from build123d import *

# Parameters (mm, degrees)
EXTRUDE_1_DEPTH          = 50
SHELL_1_T                = -1.5
CUT_EXTRUDE_1_DEPTH      = 156.758548301
CUT_EXTRUDE_1_DEPTH_BACK = 156.758548301
SKETCH_4_R               = 3.6
SKETCH_4_R_2             = 1.6
CUT_EXTRUDE_2_REACH      = 189.083
SKETCH_6_R               = 6
SKETCH_7_R               = 1.6
CUT_EXTRUDE_3_DEPTH      = 156.758548301


with BuildPart() as part:
    # 草圖3 → 填料-伸長1 (new body)
    with BuildSketch(Plane(origin=(0, 0, 0), x_dir=(1, 0, 0), z_dir=(0, 1, 0))):
        with BuildLine():
            Line((10, 41.553121903), (90, 41.553121903))
            ThreePointArc((90, 41.553121903), (97.071067812, 38.624189715), (100, 31.553121903))
            Line((100, 31.553121903), (100, -98.446878097))
            ThreePointArc((100, -98.446878097), (97.071067812, -105.517945908), (90, -108.446878097))
            Line((90, -108.446878097), (10, -108.446878097))
            ThreePointArc((10, -108.446878097), (2.928932188, -105.517945908), (0, -98.446878097))
            Line((0, -98.446878097), (0, 31.553121903))
            ThreePointArc((0, 31.553121903), (2.928932188, 38.624189715), (10, 41.553121903))
        make_face()
    extrude(amount=EXTRUDE_1_DEPTH)

    # 薄殼1
    shell_1_openings = [part.faces().sort_by_distance(p)[0] for p in [
        (50, 50, 33.446878097),
    ]]
    offset(amount=SHELL_1_T, openings=shell_1_openings, kind=Kind.INTERSECTION)

    # 草圖4 → 除料-伸長1 (cut, two sides: drawn at the far end of the back side and taken through both)
    with BuildSketch(Plane.ZY.offset(-CUT_EXTRUDE_1_DEPTH_BACK)):
        with Locations((-6.553121903, 17)):
            Circle(SKETCH_4_R)
        with Locations((73.446878097, 17)):
            Circle(SKETCH_4_R)
        with Locations((-6.552300072, 25.5)):
            Circle(SKETCH_4_R_2)
        with Locations((-6.552300072, 8.5)):
            Circle(SKETCH_4_R_2)
        with Locations((73.447699928, 25.5)):
            Circle(SKETCH_4_R_2)
        with Locations((73.447699928, 8.5)):
            Circle(SKETCH_4_R_2)
    extrude(amount=CUT_EXTRUDE_1_DEPTH + CUT_EXTRUDE_1_DEPTH_BACK, mode=Mode.SUBTRACT)

    # 草圖6 → 除料-伸長2 (cut, up to next)
    with BuildSketch(Plane.XY.offset(108.446878097), mode=Mode.PRIVATE) as cut_extrude_2_sk1:
        with Locations((50, 35)):
            Circle(SKETCH_6_R)
    cut_extrude_2_tool1 = extrude(cut_extrude_2_sk1.sketch, amount=-CUT_EXTRUDE_2_REACH, mode=Mode.PRIVATE) & part.part
    # 草圖6 → 除料-伸長2 (cut, up to next)
    with BuildSketch(Plane.XY.offset(108.446878097), mode=Mode.PRIVATE) as cut_extrude_2_sk2:
        with Locations((50, 15)):
            Circle(SKETCH_6_R)
    cut_extrude_2_tool2 = extrude(cut_extrude_2_sk2.sketch, amount=-CUT_EXTRUDE_2_REACH, mode=Mode.PRIVATE) & part.part
    add(cut_extrude_2_tool1.solids().sort_by_distance((50, 35, 108.446878))[0], mode=Mode.SUBTRACT)
    add(cut_extrude_2_tool2.solids().sort_by_distance((50, 15, 108.446878))[0], mode=Mode.SUBTRACT)

    # 草圖7 → 除料-伸長3 (cut, through all)
    with BuildSketch(Plane(origin=(100, 0, 0), x_dir=(0, 0, -1), z_dir=(1, 0, 0))):
        with Locations((-88.446878097, 46)):
            Circle(SKETCH_7_R)
        with Locations((21.553121903, 46)):
            Circle(SKETCH_7_R)
    extrude(amount=-CUT_EXTRUDE_3_DEPTH, mode=Mode.SUBTRACT)


solid = part.part
For this review, take the finished solid that the model builds, in its own axes (mm). A direction names the side the tool comes from. Give positions to 0.01 mm unless a question says otherwise; leave off trailing zeros. Loops run counter-clockwise (first coordinate to the right, second up) from the corner with the lowest first, then second, coordinate; pieces in that order, holes last. Notation, with made-up numbers: M 4,50 L 47,50 A31 cw 47,89 Z; hole C 50,-0.5 d3. An arc over 180 degrees is marked long. Answer as a JSON object with one key per item and string values. Group by question number.
Q1. For probe 1 along Z at (x, y) = (25, 24.5); probe 2 along X at (y, z) = (15.5, 32.5); probe 3 along Y at (x, z) = (30.5, 61), list the stretches that pass through material, from the lowest coordinate up. Write a range as [from, to].
Q2. Mouldability with a two-part tool opening along Y and no side actions: class faces 1 (the cylindrical face through (99.26, 45.03, 89.72)), 2 (the cylindrical face through (2.852, 24.65, -38.546)), 3 (the flat face through (51, 1.5, 32)) as +Y half, -Y half, draft (parallel to the pull), parting line (faces both ways), or undercut.
Q3. Add section A-A on x = 50. Give the boundary of the cut face in (y, z), and give its area (4 significant figures).
Q4. Add section C-C on x = 76.5. Give the boundary of the cut face in (y, z), and give its area (4 significant figures).
Q5. Add section B-B on z = -0.5. Give the boundary of the cut face in (x, y).
Q6. Add section D-D on y = 17. Give the number of separate pieces and of enclosed holes in the cut face, and give its area (3 significant figures).
Q7. Tool access review of faces 4 (the cylindrical face through (95.944, 25.41, -37.629)), 5 (the cylindrical face through (44, 15, 108)), 6 (the cylindrical face through (99.261, 13.486, -7.334)): name each direction out of +Z, -Z, +X, -X, +Y, -Y from which nothing blocks a thin tool from reaching the whole face with its end or side.
Q8. Insertion check: P1, Ø4, axis at x = 12, z = 12.5, coming from the +Y side. The pin has a flat end and moves straight along its axis. Give the tip position at first contact, or say it passes through.
Checked values:
{
 "1": {"probe 1": "[-41.55, -40.05], [106.95, 108.45]", "probe 2": "[0, 1.5], [98.5, 100]", "probe 3": "[0, 1.5]"},
 "2": {"face 1": "undercut", "face 2": "draft", "face 3": "+Y half"},
 "3": {"outline": "M 0,-41.55 L 50,-41.55 L 50,-40.05 L 1.5,-40.05 L 1.5,106.95 L 9,106.95 L 9,108.45 L 0,108.45 Z; M 21,106.95 L 29,106.95 L 29,108.45 L 21,108.45 Z; M 41,106.95 L 50,106.95 L 50,108.45 L 41,108.45 Z", "area": "334.5 mm²"},
 "4": {"outline": "M 0,-41.55 L 50,-41.55 L 50,-40.05 L 1.5,-40.05 L 1.5,106.95 L 50,106.95 L 50,108.45 L 0,108.45 Z", "area": "370.5 mm²"},
 "5": {"outline": "M 0,0 L 100,0 L 100,50 L 98.5,50 L 98.5,1.5 L 1.5,1.5 L 1.5,50 L 0,50 Z"},
 "6": {"separate pieces": "5", "enclosed holes": "0", "area": "657 mm²"},
 "7": {"face 4": "+Y", "face 5": "+Z", "face 6": "+X, -X"},
 "8": {"P1": "y = 1.5"}
}
